Read the model definition and answer for the solid it produces. Units are mm, in the model's axes. A direction names the side the tool comes from. Coordinates: 2 decimals unless noted, no trailing zeros. One line per question, with ' | ' between items. Start each with the question number.
1) A tool of negligible diameter and unlimited length cuts with its end or side. For faces 1 (the face through (2, -15, 0)), 2 (the face through (2.4, 29, -5)), 3 (the face through (2.6, 29, -5)), from which of +Z, -Z, +X, -X, +Y, -Y can it reach the whole face along a straight path? Write none if from no direction.
2) Given P1, Ø0.7, axis at y = 28, z = 5, coming from the +X side; P2, Ø10, axis at y = 23, z = 7, coming from the +X side; P3, Ø0.7, axis at y = 31.5, z = -5, coming from the -X side, each flat-ended and moving along its own axis, determine where each tip first touches the part or whether it passes through.
3) Consider probe 1 along Y at (x, z) = (2.95, -8); probe 2 along Y at (x, z) = (2.2, 4). Determine where each line is inside the solid, lowest interval first.
from build123d import *

# Parameters (mm, degrees)
SKETCH1_W                = 20
SKETCH1_H                = 30
BOSS_EXTRUDE1_DEPTH      = 5
BOSS_EXTRUDE2_DEPTH      = 10
BOSS_EXTRUDE2_DEPTH_BACK = 10
BOSS_EXTRUDE3_DEPTH      = 0.1
BOSS_EXTRUDE3_DEPTH_BACK = 0.1
SKETCH4_W                = 1.400067445
SKETCH4_H                = 17.511954704


with BuildPart() as part:
    # Sketch1 → Boss-Extrude1 (new body)
    with BuildSketch(Plane(origin=(0, 0, 0), x_dir=(0, 0, -1), z_dir=(1, 0, 0))):
        Rectangle(SKETCH1_W, SKETCH1_H)
    extrude(amount=BOSS_EXTRUDE1_DEPTH)

    # Sketch3 → Boss-Extrude2 (add, two sides: drawn at the far end of the back side and taken through both)
    with BuildSketch(Plane.XY.offset(-BOSS_EXTRUDE2_DEPTH_BACK)):
        with BuildLine():
            Line((0, 15), (5, 15))
            add(Edge.make_bspline(
                [(2.5, 22.997947181), (3.336578347, 22.9995894), (5.005761453, 20.548525939), (5, 15)],
                knots=[0, 0, 0, 0, 1, 1, 1, 1], degree=3))
            add(Edge.make_bspline(
                [(2.5, 22.997947181), (1.663421653, 22.9995894), (-0.005761453, 20.548525939), (0, 15)],
                knots=[0, 0, 0, 0, 1, 1, 1, 1], degree=3))
        make_face()
    extrude(amount=BOSS_EXTRUDE2_DEPTH + BOSS_EXTRUDE2_DEPTH_BACK)

    # Sketch4 → Boss-Extrude3 (add, two sides: drawn at the far end of the back side and taken through both)
    with BuildSketch(Plane(origin=(2.5, 0, 0), x_dir=(0, 0, -1), z_dir=(1, 0, 0)).offset(-BOSS_EXTRUDE3_DEPTH_BACK)):
        with Locations((4.675225217, 25.800434354)):
            Rectangle(SKETCH4_W, SKETCH4_H)
        with Locations((-4.675225217, 25.800434354)):
            Rectangle(SKETCH4_W, SKETCH4_H)
    extrude(amount=BOSS_EXTRUDE3_DEPTH + BOSS_EXTRUDE3_DEPTH_BACK)


solid = part.part
Report:
1) face 1: +Z, -Z, +X, -X, -Y | face 2: +Z, -Z, -X, +Y | face 3: +Z, -Z, +X, +Y
2) P1: stops at x = 2.6 | P2: stops at x = 4.82 | P3: stops at x = 2.4
3) probe 1: y = -15 to 22.81 | probe 2: y = -15 to 22.91
